Autodesk Inventor part; units mm, degrees
ref_plane "YZ Plane" through (0, 0, 0) normal (1, 0, 0) x (0, 1, 0)
ref_plane "XZ Plane" through (0, 0, 0) normal (0, 1, 0) x (-1, 0, 0)
ref_plane "XY Plane" through (0, 0, 0) normal (0, 0, 1) x (1, 0, 0)
sketch "Эскиз1" plane through (0, 0, 0) normal (0, 1, 0) x (-1, 0, 0)
  line L0 (0, 0) -> (-60, 0)
  line L1 (-60, 0) -> (-60, -60)
  line L2 (-60, -60) -> (0, -60)
  line L3 (0, -60) -> (0, 0)
  dimension "d0" = 60
  dimension "d1" = 60
extrude "Выдавливание1" add sketch "Эскиз1" along normal blind 20
sketch "Эскиз2" plane through (0, 20, 0) normal (0, 1, 0) x (1, 0, 0)
  line L0 (0, 0) -> (60, 0)
  line L1 (0, 0) -> (12, 0)
  line L2 (12, 0) -> (12, 60)
  line L3 (60, 60) -> (0, 60)
  line L4 (0, 60) -> (0, 0)
  line L5 (0, 60) -> (0, 0)
  dimension "d4" = 12
extrude "Выдавливание2" add sketch "Эскиз2" along normal blind 260
sketch "Эскиз3" plane through (0, 20, 0) normal (0, 1, 0) x (1, 0, 0)
  point P0 (0, 0)
  point P1 (26, 13)
  point P2 (26, 47)
  point P3 (50.2241, 13)
  point P4 (50.2241, 47)
hole "Отверстие1" at (26, 20, -13) at (26, 20, -47) at (50.2241, 20, -13) at (50.2241, 20, -47) direction (0, -1, 0) diameter 4 depth 40 tip angle 118
sketch "Эскиз4" plane through (12, 20, 0) normal (1, 0, 0) x (0, 0, -1)
  point P0 (0, -20)
  point P1 (30, 88)
  dimension "d14" = 0
extrude "Выдавливание3" [suppressed]
sketch "Эскиз5" plane through (12, 20, 0) normal (1, 0, 0) x (0, 0, -1)
  point P0 (0, -20)
sketch "Эскиз6" plane through (0, 0, 0) normal (0, 0, 1) x (1, 0, 0)
  line L0 (0, 0) -> (0, 280)
  line L1 (12, 20) -> (12, 280)
sketch "Эскиз7" plane through (60, 0, -60) normal (0, 0, -1) x (-1, 0, 0)
  point P0 (60, 0)
sketch "Эскиз8" plane through (12, 20, 0) normal (1, 0, 0) x (0, 0, -1)
  circle A0 centre (30, 80) radius 11.5
  point P0 (0, -20)
  point P1 (0, 80)
  dimension "d17" = 23
extrude "Выдавливание4" cut sketch "Эскиз8" against normal blind 100
sketch "Эскиз9" plane through (0, 0, -60) normal (-1, 0, 0) x (0, 0, 1)
  circle A0 centre (29.731, 99.8395) radius 12.5286
  point P0 (60, 0)
  point P1 (0, 80)
extrude "Выдавливание5" add sketch "Эскиз9" against normal blind 12
sketch "Эскиз10" plane through (0, 0, -60) normal (-1, 0, 0) x (0, 0, 1)
  line L0 (0, 0) -> (0, 280)
  circle A0 centre (30, 60) radius 11
  circle A1 centre (22, 80) radius 2
  circle A2 centre (38, 80) radius 2
  point P0 (60, 0)
  point P1 (0, 60)
  point P2 (0, 80)
  point P3 (30, 80)
  dimension "d22" = 22
  dimension "d23" = 4
  dimension "d24" = 4
extrude "Выдавливание6" cut sketch "Эскиз10" against normal blind 12
sketch "Эскиз11" plane through (0, 0, 0) normal (0, -1, 0) x (1, 0, 0)
  point P0 (0, 0)
fillet "Сопряжение1" radius 10 1 edges at (12, 20, -30)
sketch "Эскиз12" plane through (0, 0, -60) normal (-1, 0, 0) x (0, 0, 1)
  line L0 (0, 120) -> (60, 120)
  line L1 (60, 120) -> (60, 125)
  line L2 (60, 125) -> (0, 125)
  line L3 (0, 125) -> (0, 120)
  point P0 (60, 0)
  dimension "d28" = 60
  dimension "d29" = 5
extrude "Выдавливание7" add sketch "Эскиз12" against normal blind 50
fillet "Сопряжение2" radius 5 1 edges at (12, 125, -30)
sketch "Эскиз13" plane through (50, 125, 0) normal (0, 1, 0) x (1, 0, 0)
  circle A0 centre (-19, 30) radius 2
  point P0 (-50, 0)
  dimension "d33" = 4
extrude "Выдавливание8" cut sketch "Эскиз13" against normal blind 50
sketch "Эскиз14" plane through (0, 0, -60) normal (-1, 0, 0) x (0, 0, 1)
  line L0 (0, 0) -> (0, 280)
  line L1 (0, 145) -> (60, 145)
  line L2 (60, 145) -> (60, 150)
  line L3 (60, 150) -> (0, 150)
  line L4 (0, 150) -> (0, 145)
  point P0 (60, 0)
  dimension "d36" = 60
  dimension "d37" = 5
extrude "Выдавливание9" add sketch "Эскиз14" against normal blind 50
fillet "Сопряжение3" radius 5 1 edges at (12, 150, -30)
sketch "Эскиз15" plane through (12, 145, -60) normal (0, -1, 0) x (1, 0, 0)
  circle A0 centre (19, 30) radius 2
  circle A1 centre (19, 30) radius 2
  circle A2 centre (19, 30) radius 2
  point P0 (-12, 60)
  point P1 (3.4297, 11.4015)
  dimension "d41" = 4
extrude "Выдавливание10" cut sketch "Эскиз15" against normal blind 50
sketch "Эскиз16" plane through (0, 0, -60) normal (-1, 0, 0) x (0, 0, 1)
  line L0 (0, 0) -> (0, 280)
  circle A0 centre (30, 215) radius 0.5
  point P0 (60, 0)
  point P1 (0, 215)
  point P2 (0, 215)
  dimension "d44" = 1
extrude "Выдавливание11" cut sketch "Эскиз16" against normal blind 100
sketch "Эскиз17" plane through (12, 280, 0) normal (1, 0, 0) x (0, 0, -1)
  point P0 (0, -280)
sketch "Эскиз18" plane through (12, 280, 0) normal (1, 0, 0) x (0, 0, -1)
  line L0 (0, -125) -> (0, 0)
  line L1 (60, -280) -> (60, 0)
  line L2 (0, -80) -> (0, -50)
  line L3 (0, -50) -> (5, -50)
  line L4 (5, -50) -> (5, -80)
  line L5 (5, -80) -> (0, -80)
  line L6 (0, -80) -> (0, -50)
  point P0 (0, -280)
  point P1 (30, -80)
  point P2 (30, -50)
  dimension "d47" = 5
extrude "Выдавливание12" add sketch "Эскиз18" along normal blind 44.5
sketch "Эскиз19" plane through (0, 0, 0) normal (0, 0, 1) x (1, 0, 0)
  circle A0 centre (52.5, 223) radius 2
  circle A1 centre (52.5, 207) radius 2
  point P0 (0, 0)
  point P1 (52.5, 215)
  dimension "d50" = 4
  dimension "d51" = 4
extrude "Выдавливание13" cut sketch "Эскиз19" against normal blind 45
fillet "Сопряжение4" radius 10 1 edges at (12, 215, -5)
sketch "Эскиз20" plane through (12, 280, 0) normal (1, 0, 0) x (0, 0, -1)
  line L0 (0, -280) -> (0, 0)
  line L1 (0, -50.033) -> (60, -50.033)
  line L2 (60, -280) -> (60, 0)
  line L3 (60, -50.033) -> (60, 0)
  line L4 (60, 0) -> (0, 0)
  line L5 (0, 0) -> (0, -50.033)
extrude "Выдавливание14" cut sketch "Эскиз20" against normal blind 100
sketch "Эскиз21" plane through (0, 0, 0) normal (0, 0, 1) x (1, 0, 0)
  line L0 (22, 230) -> (12, 230)
  line L1 (22, 200) -> (56.5, 200)
  line L2 (12, 230) -> (56.5, 230)
  line L3 (56.5, 230) -> (56.5, 200)
  line L4 (56.5, 200) -> (12, 200)
  line L5 (12, 200) -> (12, 230)
  point P0 (0, 0)
extrude "Выдавливание15" cut sketch "Эскиз21" against normal blind 100
sketch "Эскиз22" plane through (0, 0, -60) normal (-1, 0, 0) x (0, 0, 1)
  circle A0 centre (22, 80) radius 2
  line L0 (60, 0) -> (60, 229.967)
  line L1 (0, 0) -> (0, 229.967)
  line L2 (0, 30) -> (0, 120)
  line L3 (0, 78) -> (60, 78)
  line L4 (60, 155) -> (60, 229.967)
  line L5 (60, 78) -> (60, 229.967)
  line L6 (60, 229.967) -> (0, 229.967)
  line L7 (0, 78) -> (0, 229.967)
extrude "Выдавливание16" cut sketch "Эскиз22" against normal blind 100
properties part number "Подпора"
The listing builds one solid part. Answer for the finished solid, in the listing's coordinates (mm). A direction names the side the tool comes from. Round coordinates to 2 decimals unless told otherwise and drop trailing zeros. Loops run counter-clockwise (first coordinate to the right, second up) from the corner with the lowest first, then second, coordinate; pieces in that order, holes last.
1) Given P1, Ø2.5, axis at x = 26, z = -13, coming from the +Y side; P2, Ø4.5, axis at x = 50.22, z = -47, coming from the +Y side; P3, Ø4, axis at y = 26.5, z = -27, coming from the +X side; P4, Ø24, axis at y = 63, z = -41, coming from the +X side, each flat-ended and moving along its own axis, determine where each tip first touches the part or whether it passes through.
Outcome:
P1: passes through
P2: stops at y = 20
P3: stops at x = 13.65
P4: stops at x = 12
2) A cutting plane is placed at C-C on z = -30. Determine the outline of the cut face in (x, y), plus the area to 3 significant figures.
Outcome:
outline: (0, 0) - (60, 0) - (60, 20) - (22, 20) arc R10 cw to (12, 30) - (12, 49) - (0, 49) - close; (0, 71) - (12, 71) - (12, 78) - (0, 78) - close
area: 1,650 mm2
3) A cutting plane is placed at B-B on z = -47. Determine the outline of the cut face in (x, y), plus the area to 3 significant figures.
Outcome:
outline: (0, 0) - (24, 0) - (24, 20) - (22, 20) arc R10 cw to (12, 30) - (12, 78) - (0, 78) - close; (28, 0) - (48.22, 0) - (48.22, 20) - (28, 20) - close; (52.22, 0) - (60, 0) - (60, 20) - (52.22, 20) - close
area: 1,760 mm2
4) A cutting plane is placed at A-A on y = 60. Determine the outline of the cut face in (x, z), plus the area to 3 significant figures.
Outcome:
outline: (0, -60) - (12, -60) - (12, -41) - (0, -41) - close; (0, -19) - (12, -19) - (12, 0) - (0, 0) - close
area: 456 mm2
5) Consider line 1 (X direction, y = 15, z = -13); line 2 (Y direction, x = 2, z = -30); line 3 (Y direction, x = 52, z = -49.5). Determine where each line is inside the solid, lowest interval first.
Outcome:
line 1: x = 0 to 24, 28 to 48.22, 52.22 to 60
line 2: y = 0 to 49, 71 to 78
line 3: y = 0 to 20
6) For faces 4 (the face through (28, 10, -47)), 5 (the face through (41, 20, -30)), determine the directions among +Z, -Z, +X, -X, +Y, -Y from which every point of the face is accessible in a straight line to the end or side of a thin tool.
Outcome:
face 4: +Y, -Y
face 5: +Z, -Z, +X, +Y
7) A cutting plane is placed at D-D on x = 11. Determine the outline of the cut face in (y, z).
Outcome:
outline: (0, -60) - (78, -60) - (78, 0) - (0, 0) - close; hole circle Ø22 at (60, -30)
8) For a pull along Z with two mould halves and no side action, classify faces 1 (the face through (6, 78, -30)), 2 (the face through (16, 21, 0)), 3 (the face through (27.2, 9.9, -14.6)) as released by +Z, released by -Z, zero draft, split by the parting line, or undercut.
Outcome:
face 1: zero draft
face 2: released by +Z
face 3: undercut
